Geometry: final body of the model. Coordinates: model frame, mm. Face numbers are marked on the shaded views. Give positions to 0.01 mm unless a question says otherwise; leave off trailing zeros. Order: outer loops, then holes, each group sorted by start corner. A loop starts at its lowest first (then second) coordinate and runs counter-clockwise, first axis right, second up. Notation, with made-up numbers: (57.25, -20.75) -> (98.25, -20.75) arc R22 cw to (98.25, 1.25) -> close; hole circle Ø2 at (68.5, 0). An arc over 180 degrees is marked (long way). One line per question, with ' | ' between items.
from build123d import *

# Parameters (mm, degrees)
SKETCH2_W      = 0.889
SKETCH2_H      = 1.64826619
EXTRUDE1_DEPTH = 1.905
SKETCH3_W      = 0.889
SKETCH3_H      = 2.39619966
EXTRUDE2_DEPTH = 1.905
CHAMFER1_SIZE  = 0.254


with BuildPart() as part:
    # Sketch1 → Revolve1 (revolve)
    with BuildSketch(Plane.XY):
        with BuildLine():
            Line((0, 0), (0, -11.5))
            Line((0, -11.5), (1.5, -11.5))
            Line((1.5, -11.5), (1.5, -2.25))
            Line((1.5, -2.25), (2.5, -2.25))
            Line((2.5, -2.25), (2.5, -0.75))
            ThreePointArc((2.5, -0.75), (1.305038314, -0.191538955), (0, 0))
        make_face()
    revolve(axis=Axis((0, 0, 0), (0, -1, 0)))

    # Sketch2 → Extrude1 (cut, symmetric)
    with BuildSketch(Plane.XY):
        with Locations((0, 0.074133095)):
            Rectangle(SKETCH2_W, SKETCH2_H)
    extrude(amount=EXTRUDE1_DEPTH, both=True, mode=Mode.SUBTRACT)

    # Sketch3 → Extrude2 (cut, symmetric)
    with BuildSketch(Plane(origin=(0, 0, 0), x_dir=(0, 0, -1), z_dir=(1, 0, 0))):
        with Locations((0, 0.44809983)):
            Rectangle(SKETCH3_W, SKETCH3_H)
    extrude(amount=EXTRUDE2_DEPTH, both=True, mode=Mode.SUBTRACT)

    # Chamfer1
    chamfer1_edges = [part.edges().sort_by_distance(p)[0] for p in [
        (-1.5, -11.5, 0),
    ]]
    chamfer(chamfer1_edges, length=CHAMFER1_SIZE)


solid = part.part
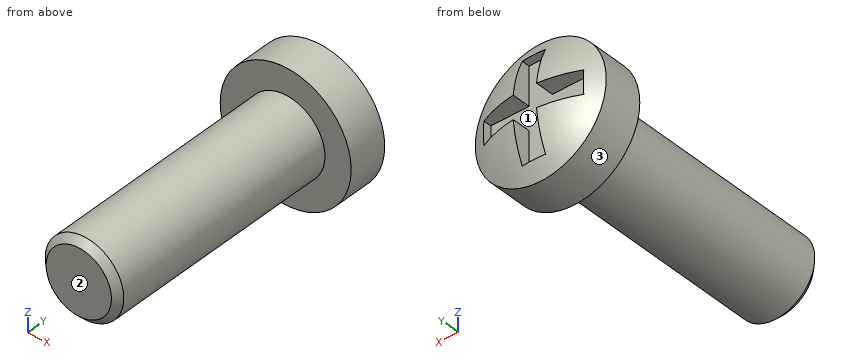
1) Material intervals for probe 1 along Y at (x, z) = (-1.55, -0.05); probe 2 along Y at (x, z) = (-0.85, 0.4); probe 3 along X at (y, z) = (-1.75, 0.1), sorted ascending. Write a range as from..to.
Check result:
probe 1: y = -2.25..-0.75 | probe 2: y = -11.5..-0.75 | probe 3: x = -2.5..2.5
2) Contact query for flat-ended pins moving along their axis: pin 1 Ø0.8 at (x, y) = (1, -0.5) entering from -Z; pin 2 Ø3 at (x, y) = (0.5, -9.5) entering from -Z; pin 3 Ø0.8 at (y, z) = (-0.5, -1) entering from -X. Output: stop coordinate, or through.
Check result:
pin 1: stops at z = -2.4 | pin 2: stops at z = -1.5 | pin 3: stops at x = -2.4
3) Section A-A on z = 0. Return loops of the section in (x, y) (3 decimals), plus the area to 3 significant figures.
Check result:
outline: (-2.5, -2.25) -> (-1.5, -2.25) -> (-1.5, -11.246) -> (-1.246, -11.5) -> (1.246, -11.5) -> (1.5, -11.246) -> (1.5, -2.25) -> (2.5, -2.25) -> (2.5, -0.75) arc R4.542 ccw to (1.905, -0.419) -> (1.905, -0.75) -> (-1.905, -0.75) -> (-1.905, -0.419) arc R4.542 ccw to (-2.5, -0.75) -> close | area: 35.4 mm^2
4) Section B-B on x = 0. Return loops of the section in (y, z) (3 decimals).
Check result:
outline: (-11.5, -1.246) -> (-11.246, -1.5) -> (-2.25, -1.5) -> (-2.25, -2.5) -> (-0.75, -2.5) arc R4.542 ccw to (-0.419, -1.905) -> (-0.75, -1.905) -> (-0.75, 1.905) -> (-0.419, 1.905) arc R4.542 ccw to (-0.75, 2.5) -> (-2.25, 2.5) -> (-2.25, 1.5) -> (-11.246, 1.5) -> (-11.5, 1.246) -> close
5) Pull-direction query (Z, two-part tool) for the marked faces 1, 2 and 3; classes: +Z half, -Z half, draft (parallel to the pull), parting line (faces both ways), or undercut.
Check result:
face 1: undercut | face 2: draft | face 3: parting line
6) Section C-C on y = -5. Return loops of the section in (x, z).
Check result:
outline: circle Ø3 at (0, 0)
7) Section D-D on z = -1.7. Return loops of the section in (x, y), plus the area to 3 significant figures.
Check result:
outline: (-1.83, -2.25) -> (1.83, -2.25) -> (1.83, -0.75) arc R4.21 ccw to (0.44, -0.35) -> (0.44, -0.75) -> (-0.44, -0.75) -> (-0.44, -0.35) arc R4.21 ccw to (-1.83, -0.75) -> close | area: 6.17 mm^2
